Autodesk Inventor part; units mm, degrees
ref_plane "YZ Plane" through (0, 0, 0) normal (1, 0, 0) x (0, 1, 0)
ref_plane "XZ Plane" through (0, 0, 0) normal (0, 1, 0) x (-1, 0, 0)
ref_plane "XY Plane" through (0, 0, 0) normal (0, 0, 1) x (1, 0, 0)
sketch "Sketch1" plane through (0, 0, 0) normal (1, 0, 0) x (0, 1, 0)
  line L0 (11.1495, -7.3) -> (-11.1495, -7.3)
  line L1 (-11.1495, -7.3) -> (-11.1495, -5.7)
  line L2 (-11.1495, -5.7) -> (11.1495, -5.7)
  line L3 (11.1495, -5.7) -> (11.1495, -7.3)
  line L4 (11.1495, -7.3) -> (-11.1495, -5.7) construction
  line L5 (-11.1495, -7.3) -> (11.1495, -5.7) construction
  point P0 (0, 0)
  point P1 (0, -6.5)
  dimension "d1" = 22.299
  dimension "d2" = 1.6
extrude "Extrusion1" add sketch "Sketch1" along normal mid plane 22
sketch "Sketch2" plane through (-11, -11.1495, -5.7) normal (0, 0, 1) x (1, 0, 0)
  line L0 (11.7587, 9.6495) -> (16.7587, 9.6495)
  line L1 (16.7587, 9.6495) -> (16.7587, 12.6495)
  line L2 (16.7587, 12.6495) -> (11.7587, 12.6495)
  line L3 (11.7587, 15.6495) -> (11.7587, 6.6495)
  line L4 (11.7587, 11.1495) -> (4.7587, 11.1495) construction
  line L5 (4.7587, 11.1495) -> (11.7587, 6.6495)
  line L6 (4.7587, 11.1495) -> (11.7587, 15.6495)
  line L7 (16.7587, 11.1495) -> (18.5587, 11.1495) construction
  line L8 (0, 22.299) -> (0, 0)
  point P0 (11.7587, 11.1495)
  point P1 (11.7587, 12.6495)
  dimension "d6" = 3
  dimension "d9" = 9
  dimension "d10" = 7
  dimension "d11" = 5
  dimension "d14" = 5
extrude "Extrusion2" cut sketch "Sketch2" against normal blind 1
equation "\"d14\" = d11"
properties part number "Part2_3DPrint"
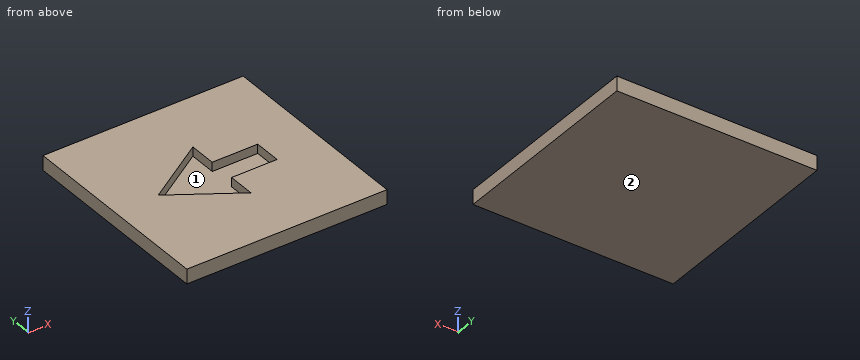
Design review of the part built by this model. Coordinates are the model's own, in mm. Face numbers are marked on the shaded views. Coordinates: 2 decimals unless noted, no trailing zeros. Loops run counter-clockwise (first coordinate to the right, second up) from the corner with the lowest first, then second, coordinate; pieces in that order, holes last. Notation, with made-up numbers: (-10.5, 32) - (37.5, 32) arc R26 cw to (37.5, 66) - close; hole circle Ø3 at (60, 2.25). An arc over 180 degrees is marked (long way). Use CSV: the item, a comma, the result in double quotes. Start each with the question number.
1) Consider section A-A on z = -6.35. Write out the cut boundary in (x, y).
2) Consider section B-B on x = 4.5. Write out the cut boundary in (y, z), then the cut area to 3 significant figures.
3) Consider section C-C on y = -0.5. Write out the cut boundary in (x, z), then the cut area to 3 significant figures.
4) The part is to be moulded in two halves that separate along Y. For the marked faces 1 and 2, say which applies: +Y half, -Y half, draft (parallel to the pull), parting line (faces both ways), or undercut.
5) Wall thickness on L1, parallel to Y at x = 1.75, z = -6.2; L2, parallel to Z at x = 0.5, y = -4.25; L3, parallel to X at y = 1.75, z = -6.4: over which ranges is each line inside the solid? List them lowest first. Write a range as from..to.
Geometry says:
1,outline,"(-11, -11.15) - (11, -11.15) - (11, 11.15) - (-11, 11.15) - close; hole (-6.24, 0) - (0.76, -4.5) - (0.76, -1.5) - (5.76, -1.5) - (5.76, 1.5) - (0.76, 1.5) - (0.76, 4.5) - close"
2,outline,"(-11.15, -7.3) - (11.15, -7.3) - (11.15, -5.7) - (1.5, -5.7) - (1.5, -6.7) - (-1.5, -6.7) - (-1.5, -5.7) - (-11.15, -5.7) - close"
2,area,"32.7 mm^2"
3,outline,"(-11, -7.3) - (11, -7.3) - (11, -5.7) - (5.76, -5.7) - (5.76, -6.7) - (-5.46, -6.7) - (-5.46, -5.7) - (-11, -5.7) - close"
3,area,"24.0 mm^2"
4,face 1,"undercut"
4,face 2,"draft"
5,L1,"-11.15..-1.5, 1.5..11.15"
5,L2,"-7.3..-6.7"
5,L3,"-11..-3.52, 0.76..11"
